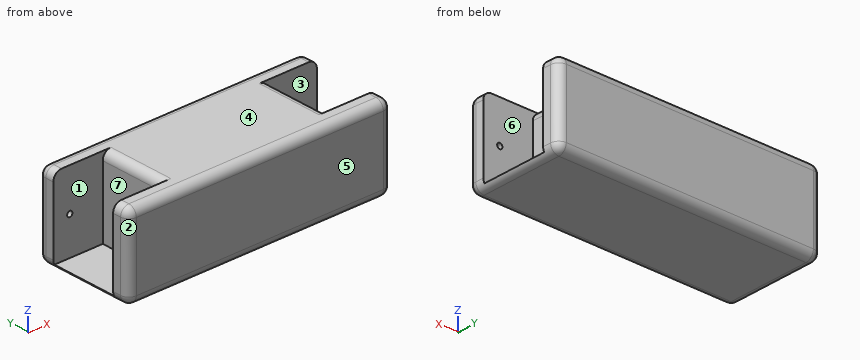
```python
from build123d import *

# Parameters (mm, degrees)
SKETCH2_W           = 160
SKETCH2_H           = 60
BOSS_EXTRUDE1_DEPTH = 50
SKETCH4_W           = 30
SKETCH4_H           = 40
CUT_EXTRUDE1_DEPTH  = 99.994949366
SKETCH5_R           = 1.6
CUT_EXTRUDE2_DEPTH  = 3.2
CUT_EXTRUDE3_START  = -3.2
SKETCH6_R           = 1.6
CUT_EXTRUDE3_DEPTH  = 3.2
CUT_EXTRUDE5_START  = -6.8
SKETCH7_R           = 1.6
CUT_EXTRUDE5_DEPTH  = 3.2
CUT_EXTRUDE6_START  = -10
SKETCH8_R           = 1.6
CUT_EXTRUDE6_DEPTH  = 3.2
SKETCH9_W           = 2.5
SKETCH9_H           = 40
BOSS_EXTRUDE2_DEPTH = 30
SKETCH10_W          = 2.5
SKETCH10_H          = 40
BOSS_EXTRUDE3_DEPTH = 30
FILLET1_R           = 5


with BuildPart() as part:
    # Sketch2 → Boss-Extrude1 (new body)
    with BuildSketch(Plane.XY):
        Rectangle(SKETCH2_W, SKETCH2_H)
    extrude(amount=BOSS_EXTRUDE1_DEPTH)

    # Sketch4 → Cut-Extrude1 (cut, through all)
    with BuildSketch(Plane.XY.offset(50)):
        with Locations((65, 0)):
            Rectangle(SKETCH4_W, SKETCH4_H)
        with Locations((-65, 0)):
            Rectangle(SKETCH4_W, SKETCH4_H)
    extrude(amount=-CUT_EXTRUDE1_DEPTH, mode=Mode.SUBTRACT)

    # Sketch5 → Cut-Extrude2 (cut)
    with BuildSketch(Plane(origin=(0, 20, 0), x_dir=(-1, 0, 0), z_dir=(0, -1, 0))):
        with Locations(Location((70, -25, 0), (0, 0, 90))):
            Circle(SKETCH5_R)
    extrude(amount=-CUT_EXTRUDE2_DEPTH, mode=Mode.SUBTRACT)

    # Sketch6 → Cut-Extrude3 (cut)
    with BuildSketch(Plane(origin=(0, -20, 0), x_dir=(1, 0, 0), z_dir=(0, 1, 0)).offset(CUT_EXTRUDE3_START)):
        with Locations(Location((-70, -25, 0), (0, 0, 90))):
            Circle(SKETCH6_R)
    extrude(amount=CUT_EXTRUDE3_DEPTH, mode=Mode.SUBTRACT)

    # Sketch7 → Cut-Extrude5 (cut)
    with BuildSketch(Plane(origin=(0, 30, 0), x_dir=(1, 0, 0), z_dir=(0, 1, 0)).offset(CUT_EXTRUDE5_START)):
        with Locations(Location((70, -25, 0), (0, 0, 270))):
            Circle(SKETCH7_R)
    extrude(amount=-CUT_EXTRUDE5_DEPTH, mode=Mode.SUBTRACT)

    # Sketch8 → Cut-Extrude6 (cut)
    with BuildSketch(Plane.XZ.offset(30).offset(CUT_EXTRUDE6_START)):
        with Locations(Location((70, 25, 0), (0, 0, 90))):
            Circle(SKETCH8_R)
    extrude(amount=CUT_EXTRUDE6_DEPTH, mode=Mode.SUBTRACT)

    # Sketch9 → Boss-Extrude2 (add)
    with BuildSketch(Plane.ZY.offset(50)):
        with Locations((1.25, 0)):
            Rectangle(SKETCH9_W, SKETCH9_H)
    extrude(amount=BOSS_EXTRUDE2_DEPTH)

    # Sketch10 → Boss-Extrude3 (add)
    with BuildSketch(Plane(origin=(50, 0, 0), x_dir=(0, 0, -1), z_dir=(1, 0, 0))):
        with Locations((-1.25, 0)):
            Rectangle(SKETCH10_W, SKETCH10_H)
    extrude(amount=BOSS_EXTRUDE3_DEPTH)

    # Fillet1
    # the kernel refuses this fillet: 5 mm, written as the material it takes off along each edge
    with BuildSketch(Plane(origin=(-75, -25, 45), x_dir=(0, -1, 0), z_dir=(0, 0, 1))) as fillet1_piece_1_section:
        Polygon((0, 0), (FILLET1_R, 0), (FILLET1_R, -FILLET1_R), (0, -FILLET1_R), align=None)
    fillet1_piece_1 = extrude(amount=FILLET1_R, mode=Mode.PRIVATE)
    fillet1_piece_1 = fillet1_piece_1 - Plane(origin=(-75, -25, 45), x_dir=(0.7071067811865475, 0.7071067811865475, 0), z_dir=(0, 0, 1)) * Sphere(FILLET1_R, mode=Mode.PRIVATE)
    add(fillet1_piece_1, mode=Mode.SUBTRACT)
    with BuildSketch(Plane(origin=(-75, 25, 45), x_dir=(0, 0, 1), z_dir=(0, 1, 0))) as fillet1_piece_2_section:
        Polygon((0, 0), (FILLET1_R, 0), (FILLET1_R, -FILLET1_R), (0, -FILLET1_R), align=None)
    fillet1_piece_2 = extrude(amount=FILLET1_R, mode=Mode.PRIVATE)
    fillet1_piece_2 = fillet1_piece_2 - Plane(origin=(-75, 25, 45), x_dir=(0.7071067811865475, 0, -0.7071067811865475), z_dir=(0, 1, 0)) * Sphere(FILLET1_R, mode=Mode.PRIVATE)
    add(fillet1_piece_2, mode=Mode.SUBTRACT)
    with BuildSketch(Plane(origin=(75, 25, 45), x_dir=(0, 0, 1), z_dir=(0, 1, 0))) as fillet1_piece_3_section:
        Polygon((0, 0), (FILLET1_R, 0), (FILLET1_R, FILLET1_R), (0, FILLET1_R), align=None)
    fillet1_piece_3 = extrude(amount=FILLET1_R, mode=Mode.PRIVATE)
    fillet1_piece_3 = fillet1_piece_3 - Plane(origin=(75, 25, 45), x_dir=(-0.7071067811865475, 0, -0.7071067811865475), z_dir=(0, 1, 0)) * Sphere(FILLET1_R, mode=Mode.PRIVATE)
    add(fillet1_piece_3, mode=Mode.SUBTRACT)
    with BuildSketch(Plane(origin=(75, -25, 45), x_dir=(0, -1, 0), z_dir=(0, 0, 1))) as fillet1_piece_4_section:
        Polygon((0, 0), (FILLET1_R, 0), (FILLET1_R, FILLET1_R), (0, FILLET1_R), align=None)
    fillet1_piece_4 = extrude(amount=FILLET1_R, mode=Mode.PRIVATE)
    fillet1_piece_4 = fillet1_piece_4 - Plane(origin=(75, -25, 45), x_dir=(-0.7071067811865476, 0.7071067811865475, 0), z_dir=(0, 0, 1)) * Sphere(FILLET1_R, mode=Mode.PRIVATE)
    add(fillet1_piece_4, mode=Mode.SUBTRACT)
    with BuildSketch(Plane(origin=(75, -25, 5), x_dir=(0, 0, -1), z_dir=(0, -1, 0))) as fillet1_piece_5_section:
        Polygon((0, 0), (FILLET1_R, 0), (FILLET1_R, FILLET1_R), (0, FILLET1_R), align=None)
    fillet1_piece_5 = extrude(amount=FILLET1_R, mode=Mode.PRIVATE)
    fillet1_piece_5 = fillet1_piece_5 - Plane(origin=(75, -25, 5), x_dir=(-0.7071067811865475, 0, 0.7071067811865475), z_dir=(0, -1, 0)) * Sphere(FILLET1_R, mode=Mode.PRIVATE)
    add(fillet1_piece_5, mode=Mode.SUBTRACT)
    with BuildSketch(Plane(origin=(75, 25, 5), x_dir=(0, 0, -1), z_dir=(0, 1, 0))) as fillet1_piece_6_section:
        Polygon((0, 0), (FILLET1_R, 0), (FILLET1_R, -FILLET1_R), (0, -FILLET1_R), align=None)
    fillet1_piece_6 = extrude(amount=FILLET1_R, mode=Mode.PRIVATE)
    fillet1_piece_6 = fillet1_piece_6 - Plane(origin=(75, 25, 5), x_dir=(-0.7071067811865475, 0, 0.7071067811865475), z_dir=(0, 1, 0)) * Sphere(FILLET1_R, mode=Mode.PRIVATE)
    add(fillet1_piece_6, mode=Mode.SUBTRACT)
    with BuildSketch(Plane(origin=(-75, 25, 5), x_dir=(0, 0, -1), z_dir=(0, 1, 0))) as fillet1_piece_7_section:
        Polygon((0, 0), (FILLET1_R, 0), (FILLET1_R, FILLET1_R), (0, FILLET1_R), align=None)
    fillet1_piece_7 = extrude(amount=FILLET1_R, mode=Mode.PRIVATE)
    fillet1_piece_7 = fillet1_piece_7 - Plane(origin=(-75, 25, 5), x_dir=(0.7071067811865475, 0, 0.7071067811865475), z_dir=(0, 1, 0)) * Sphere(FILLET1_R, mode=Mode.PRIVATE)
    add(fillet1_piece_7, mode=Mode.SUBTRACT)
    with BuildSketch(Plane(origin=(-75, -25, 5), x_dir=(0, 0, -1), z_dir=(0, -1, 0))) as fillet1_piece_8_section:
        Polygon((0, 0), (FILLET1_R, 0), (FILLET1_R, -FILLET1_R), (0, -FILLET1_R), align=None)
    fillet1_piece_8 = extrude(amount=FILLET1_R, mode=Mode.PRIVATE)
    fillet1_piece_8 = fillet1_piece_8 - Plane(origin=(-75, -25, 5), x_dir=(0.7071067811865475, 0, 0.7071067811865475), z_dir=(0, -1, 0)) * Sphere(FILLET1_R, mode=Mode.PRIVATE)
    add(fillet1_piece_8, mode=Mode.SUBTRACT)
    with BuildSketch(Plane(origin=(-80, -25, 50), x_dir=(1, 0, 0), z_dir=(0, 1, 0)), Plane(origin=(-80, 7.5, 50), x_dir=(1, 0, 0), z_dir=(0, 1, 0)), Plane(origin=(80, 25, 50), x_dir=(-1, 0, 0), z_dir=(0, -1, 0)), Plane(origin=(80, -7.5, 50), x_dir=(-1, 0, 0), z_dir=(0, -1, 0))) as fillet1_piece_9:
        with BuildLine():
            CenterArc((FILLET1_R, FILLET1_R), FILLET1_R, 180, 90)
            Line((0, FILLET1_R), (0, 0))
            Line((0, 0), (FILLET1_R, 0))
        make_face()
    extrude(amount=17.5, mode=Mode.SUBTRACT)
    with BuildSketch(Plane(origin=(50, 20, 50), x_dir=(-1, 0, 0), z_dir=(0, -1, 0)), Plane(origin=(80, 30, 5), x_dir=(-1, 0, 0), z_dir=(0, 0, 1)), Plane(origin=(-80, -30, 5), x_dir=(1, 0, 0), z_dir=(0, 0, 1))) as fillet1_piece_10:
        with BuildLine():
            CenterArc((FILLET1_R, FILLET1_R), FILLET1_R, 180, 90)
            Line((0, FILLET1_R), (0, 0))
            Line((0, 0), (FILLET1_R, 0))
        make_face()
    extrude(amount=40, mode=Mode.SUBTRACT)
    with BuildSketch(Plane(origin=(80, -30, 5), x_dir=(-1, 0, 0), z_dir=(0, 0, 1)), Plane(origin=(-80, 30, 5), x_dir=(1, 0, 0), z_dir=(0, 0, 1)), Plane(origin=(-50, 20, 50), x_dir=(1, 0, 0), z_dir=(0, -1, 0))) as fillet1_piece_11:
        with BuildLine():
            CenterArc((FILLET1_R, -FILLET1_R), FILLET1_R, 90, 90)
            Line((0, -FILLET1_R), (0, 0))
            Line((0, 0), (FILLET1_R, 0))
        make_face()
    extrude(amount=40, mode=Mode.SUBTRACT)
    with BuildSketch(Plane(origin=(80, -25, 0), x_dir=(-1, 0, 0), z_dir=(0, 1, 0)), Plane(origin=(-80, 25, 0), x_dir=(1, 0, 0), z_dir=(0, -1, 0))) as fillet1_piece_12:
        with BuildLine():
            CenterArc((FILLET1_R, FILLET1_R), FILLET1_R, 180, 90)
            Line((0, FILLET1_R), (0, 0))
            Line((0, 0), (FILLET1_R, 0))
        make_face()
    extrude(amount=50, mode=Mode.SUBTRACT)
    with BuildSketch(Plane(origin=(-75, 30, 0), x_dir=(0, 0, 1), z_dir=(1, 0, 0)), Plane(origin=(75, -30, 0), x_dir=(0, 0, 1), z_dir=(-1, 0, 0)), Plane(origin=(75, -30, 50), x_dir=(0, 1, 0), z_dir=(-1, 0, 0))) as fillet1_piece_13:
        with BuildLine():
            CenterArc((FILLET1_R, FILLET1_R), FILLET1_R, 180, 90)
            Line((0, FILLET1_R), (0, 0))
            Line((0, 0), (FILLET1_R, 0))
        make_face()
    extrude(amount=150, mode=Mode.SUBTRACT)
    with BuildSketch(Plane(origin=(-75, 30, 50), x_dir=(0, 0, -1), z_dir=(1, 0, 0))) as fillet1_piece_14:
        with BuildLine():
            CenterArc((FILLET1_R, -FILLET1_R), FILLET1_R, 90, 90)
            Line((0, -FILLET1_R), (0, 0))
            Line((0, 0), (FILLET1_R, 0))
        make_face()
    extrude(amount=150, mode=Mode.SUBTRACT)


solid = part.part
```
Geometry: final body of the model. Coordinates: model frame, mm. Face numbers are marked on the shaded views. A direction names the side the tool comes from. Round coordinates to 2 decimals unless told otherwise and drop trailing zeros. Order: outer loops, then holes, each group sorted by start corner. A loop starts at its lowest first (then second) coordinate and runs counter-clockwise, first axis right, second up. Notation, with made-up numbers: (51, 38) -> (74, 38) arc R11 ccw to (74, 57) -> close; hole circle Ø2 at (89.5, 22.25). An arc over 180 degrees is marked (long way). Use one line per item in the form item = value.
(1) First-contact query: pin 1 Ø12 at (y, z) = (-8.5, 17.5) entering from +X; pin 2 Ø2 at (y, z) = (-1, 26.5) entering from -X; pin 3 Ø12 at (x, y) = (56.5, -13) entering from +Z. Flat tips, straight axial feed; report the tip coordinate or a pass-through.
Results list:
pin_1 = 50
pin_2 = -50
pin_3 = 2.5
(2) Draft query along Y for the marked faces 4, 5, 6 and 7. Return one class per face: pulls with the +Y half, pulls with the -Y half, needs draft (parallel to the pull), parting line crosses it, or undercut.
Results list:
face_4 = needs draft
face_5 = pulls with the -Y half
face_6 = undercut
face_7 = undercut
(3) Section D-D on x = -59. Return loops of the section in (y, z), and give its area (3 significant figures).
Results list:
outline = (-30, 5) arc R5 ccw to (-25, 0) -> (25, 0) arc R5 ccw to (30, 5) -> (30, 45) arc R5 ccw to (25, 50) -> (20, 50) -> (20, 2.5) -> (-20, 2.5) -> (-20, 50) -> (-25, 50) arc R5 ccw to (-30, 45) -> close
area = 1,080 mm^2
(4) Access query for the marked faces 1, 2 and 3. Directions: +Z, -Z, +X, -X, +Y, -Y. A direction counts if a zero-diameter tool reaches every point of the face in a straight line with its end or side. Return the directions, or none.
Results list:
face_1 = +Z, -X
face_2 = +Z, -Z, -X, -Y
face_3 = +Z, +X
(5) Section A-A on x = 48. Return loops of the section in (y, z).
Results list:
outline = (-30, 5) arc R5 ccw to (-25, 0) -> (25, 0) arc R5 ccw to (30, 5) -> (30, 45) arc R5 ccw to (25, 50) -> (20, 50) -> (20, 49) -> (-20, 49) -> (-20, 50) -> (-25, 50) arc R5 ccw to (-30, 45) -> close
(6) Ray query, probe 1 along X at (y, z) = (21, 25); probe 2 along Z at (x, y) = (70, -22.1); probe 3 along Y at (x, z) = (72.5, 44.5). Return the intervals inside material, ascending. Write a range as [from, to].
Results list:
probe_1 = [-80, -71.6], [-68.4, 68.4], [71.6, 80]
probe_2 = [0, 23.4], [26.6, 50]
probe_3 = [-30, -20], [20, 30]
(7) Section C-C on y = -10.5. Return loops of the section in (x, z), and give its area (3 significant figures).
Results list:
outline = (-79.33, 2.5) arc R5 ccw to (-75, 0) -> (75, 0) arc R5 ccw to (79.33, 2.5) -> (50, 2.5) -> (50, 45) arc R5 ccw to (45, 50) -> (-45, 50) arc R5 ccw to (-50, 45) -> (-50, 2.5) -> close
area = 5,130 mm^2
